Source: CAD feature listing. Evaluate the final solid. Frame: model axes, mm. A direction names the side the tool comes from. Round coordinates to 2 decimals unless told otherwise and drop trailing zeros. Order: outer loops, then holes, each group sorted by start corner. A loop starts at its lowest first (then second) coordinate and runs counter-clockwise, first axis right, second up. Notation, with made-up numbers: M 72.5,45.5 L 117.5,45.5 A17 cw 117.5,57.5 Z; hole C -1,-31.5 d3. An arc over 180 degrees is marked long. Answer as CSV lines item,"result". Start each with the question number.
Item 1: Set-up query: faces 1 (the face through (0, 3, 0)), 2 (the face through (0, 0, -18)). Return all of +Z, -Z, +X, -X, +Y, -Y with unobstructed straight access to the full face (end or side cutting, diameter ignored); none if empty.
Item 2: Section query A-A on x = 0. Return the cut outline in (y, z), plus the area to 3 significant figures.
Item 3: Section query C-C on x = -4. Return the cut outline in (y, z), plus the area to 3 significant figures.
Item 4: Line query: line 1 (Z direction, x = -0.5, y = 7.5); line 2 (Z direction, x = 0.25, y = 2.75); line 3 (Y direction, x = -3, z = -4). Output: solid intervals per line, ascending. Write a range as [from, to].
Item 5: Section query B-B on y = 4.5. Return the cut outline in (x, z).
from build123d import *

# Parameters (mm, degrees)
SKETCH1_R           = 4.75
BOSS_EXTRUDE1_DEPTH = 3
BOSS_EXTRUDE2_DEPTH = 10
CUT_EXTRUDE1_DEPTH  = 7


with BuildPart() as part:
    # Sketch1 → Boss-Extrude1 (new body)
    with BuildSketch(Plane(origin=(0, 0, 0), x_dir=(1, 0, 0), z_dir=(0, 1, 0))):
        Circle(SKETCH1_R)
    extrude(amount=BOSS_EXTRUDE1_DEPTH)

    # Sketch2 → Boss-Extrude2 (add)
    with BuildSketch(Plane(origin=(0, 0, 0), x_dir=(1, 0, 0), z_dir=(0, 1, 0))):
        with BuildLine():
            Line((-4.75, 0), (-4.75, 40))
            Line((-4.75, 40), (4.75, 40))
            Line((4.75, 40), (4.75, 0))
            ThreePointArc((4.75, 0), (0, 4.75), (-4.75, 0))
        make_face()
    extrude(amount=BOSS_EXTRUDE2_DEPTH)

    # Sketch3 → Cut-Extrude1 (cut)
    with BuildSketch(Plane(origin=(0, 10, 0), x_dir=(1, 0, 0), z_dir=(0, 1, 0))):
        with BuildLine():
            ThreePointArc((-4.75, 0), (-3.358757211, 3.358757211), (0, 4.75))
            Line((0, 4.75), (-4.75, 4.75))
            Line((-4.75, 4.75), (-4.75, 0))
        make_face()
        with BuildLine():
            Line((4.75, 4.75), (0, 4.75))
            ThreePointArc((0, 4.75), (3.358757211, 3.358757211), (4.75, 0))
            Line((4.75, 0), (4.75, 4.75))
        make_face()
    extrude(amount=-CUT_EXTRUDE1_DEPTH, mode=Mode.SUBTRACT)


solid = part.part
Results:
1,face 1,"+Z, +X, -X, +Y"
1,face 2,"+Z, -Z, +X, -X, -Y"
2,outline,"M 0,-40 L 10,-40 L 10,-4.75 L 3,-4.75 L 3,4.75 L 0,4.75 Z"
2,area,"381 mm^2"
3,outline,"M 0,-40 L 10,-40 L 10,-4.75 L 3,-4.75 L 3,2.56 L 0,2.56 Z"
3,area,"374 mm^2"
4,line 1,"[-40, -4.75]"
4,line 2,"[-40, 4.74]"
4,line 3,"[0, 3]"
5,outline,"M -4.75,-40 L 4.75,-40 L 4.75,-4.75 L -4.75,-4.75 Z"
